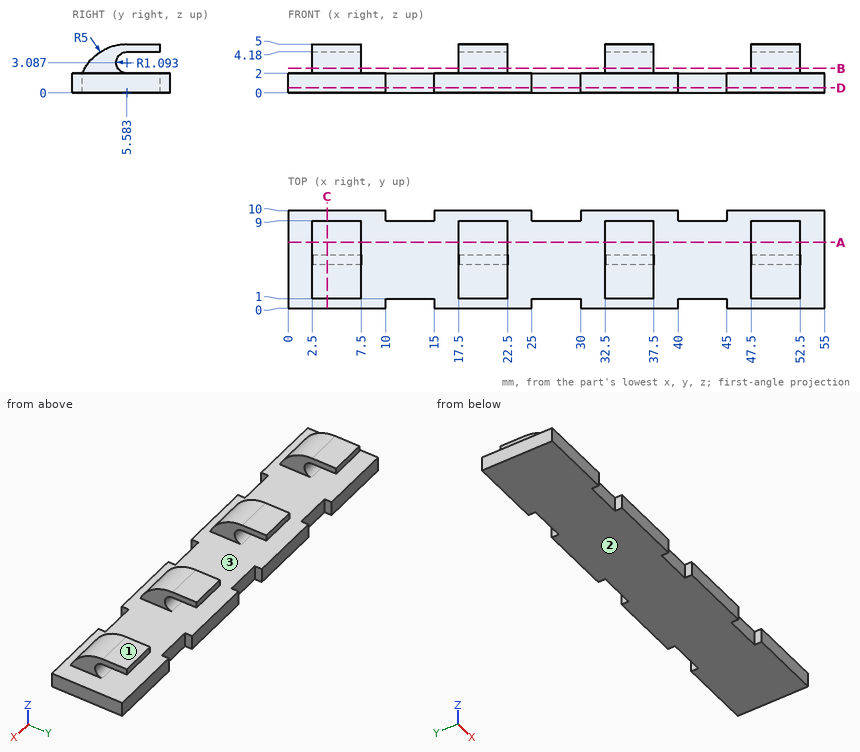
Here's the drawing with two shaded views (mm, measured from the low corner). I have some questions. Round coordinates to 2 decimals unless told otherwise and drop trailing zeros. Write each loop counter-clockwise with the first axis right and the second up, starting at its lowest first coordinate (ties: lowest second). Pieces come first, ordered by that corner, then holes. Notation, with made-up numbers: M 71,23.5 L 99,23.5 A18 ccw 99,39.5 Z; hole C -37,10 d2. An arc over 180 degrees is marked long. Answer in a Markdown table with one row per item. Add a question column.
Q1. Imagine slicing it at D-D (z = 0.5). Please give me the cut outline in (x, y).
Q2. If I drill on line 1 (X direction, y = 2.75, z = 3.35); line 2 (Z direction, x = 28, y = 8); line 3 (Y direction, x = 28, z = 0.9), over which ranges is the centre line in solid material (lowest first)? Write a range as from..to.
Q3. Will these pins go through, and if not, where does the flat tip stop? pin 1 Ø1.7 at (x, y) = (6, 7.5) entering from -Z; pin 2 Ø0.7 at (x, z) = (4, 4.5) entering from +Y; pin 3 Ø2 at (x, z) = (14.5, 4) entering from -Y; pin 4 Ø1 at (x, z) = (26.5, 0.5) entering from -Y.
Q4. Imagine slicing it at A-A (y = 6.75). Please give me the cut outline in (x, z).
Q5. If we mould it in two halves opening along Z, with no side actions, what happens to the marked faces 1, 2 and 3? For each: +Z half, -Z half, draft (parallel to the pull), parting line (faces both ways), or undercut.
Q6. Imagine slicing it at C-C (x = 4). Please give me the cut outline in (y, z).
Q7. Imagine slicing it at B-B (z = 2.5). Please give me the cut outline in (x, y).
Values:
| question | item | result |
|---|---|---|
| 1 | outline | M 0,0 L 10,0 L 10,1 L 15,1 L 15,0 L 25,0 L 25,1 L 30,1 L 30,0 L 40,0 L 40,1 L 45,1 L 45,0 L 55,0 L 55,10 L 45,10 L 45,9 L 40,9 L 40,10 L 30,10 L 30,9 L 25,9 L 25,10 L 15,10 L 15,9 L 10,9 L 10,10 L 0,10 Z |
| 2 | line 1 | 2.5..7.5, 17.5..22.5, 32.5..37.5, 47.5..52.5 |
| 2 | line 2 | 0..2 |
| 2 | line 3 | 1..9 |
| 3 | pin 1 | z = 0 |
| 3 | pin 2 | y = 9 |
| 3 | pin 3 | through |
| 3 | pin 4 | y = 1 |
| 4 | outline | M 0,0 L 55,0 L 55,2 L 0,2 Z; M 2.5,4.18 L 7.5,4.18 L 7.5,5 L 2.5,5 Z; M 17.5,4.18 L 22.5,4.18 L 22.5,5 L 17.5,5 Z; M 32.5,4.18 L 37.5,4.18 L 37.5,5 L 32.5,5 Z; M 47.5,4.18 L 52.5,4.18 L 52.5,5 L 47.5,5 Z |
| 5 | face 1 | +Z half |
| 5 | face 2 | -Z half |
| 5 | face 3 | undercut |
| 6 | outline | M 0,0 L 10,0 L 10,2 L 5.47,2 A1.09 cw 5.58,4.18 L 9,4.18 L 9,5 L 5.58,5 A5 ccw 1,2 L 0,2 Z |
| 7 | outline | M 2.5,1.25 L 7.5,1.25 L 7.5,4.66 L 2.5,4.66 Z; M 17.5,1.25 L 22.5,1.25 L 22.5,4.66 L 17.5,4.66 Z; M 32.5,1.25 L 37.5,1.25 L 37.5,4.66 L 32.5,4.66 Z; M 47.5,1.25 L 52.5,1.25 L 52.5,4.66 L 47.5,4.66 Z |
